For this review, take the finished solid that the model builds, in its own axes (mm). Face numbers are marked on the shaded views. Coordinates: 2 decimals unless noted, no trailing zeros. Return JSON: item names as keys, results as strings.
Autodesk Inventor part; units mm, degrees
ref_plane "YZ Plane" through (0, 0, 0) normal (1, 0, 0) x (0, 1, 0)
ref_plane "XZ Plane" through (0, 0, 0) normal (0, 1, 0) x (-1, 0, 0)
ref_plane "XY Plane" through (0, 0, 0) normal (0, 0, 1) x (1, 0, 0)
sketch "Sketch1" plane through (0, 0, 0) normal (0, 0, 1) x (1, 0, 0)
  circle A0 centre (0, 0) radius 23.15
  circle A1 centre (0, 0) radius 26.9875
  dimension "d0" = 46.3
  dimension "d1" = 53.975
extrude "Extrusion1" add sketch "Sketch1" along normal blind 12.7
chamfer "Chamfer1" distance 3.175 angle 45 1 edges at (-23.15, 0, 0)
sketch "Sketch2" plane through (0, 0, 0) normal (1, 0, 0) x (0, 1, 0)
  line L0 (26.9875, 0) -> (26.9875, 12.7)
  circle A0 centre (26.9875, 6.35) radius 1.5875
  line L1 (0, 0) -> (0, 25.7479) construction
  dimension "d7" = 3.175
revolve "Revolution1" cut sketch "Sketch2" angle 360 about axis through (0, 0, 0) along (0, 0, 1)
chamfer "Chamfer2" distance 1.5875 angle 45 1 edges at (-26.9875, 0, 12.7)
properties part number "Ring Hub" material "Nylon 6/6"
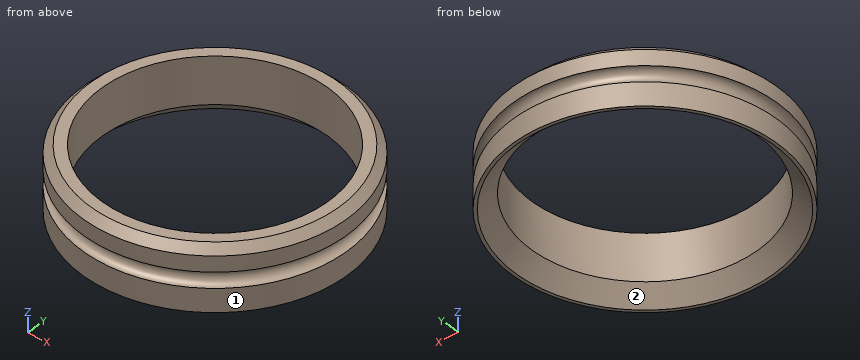
1. Clearance check with flat-ended pins moving along their axes: pin 1 Ø6 at (x, z) = (2, 2.5) entering from +Y; pin 2 Ø4 at (x, z) = (10.5, 7) entering from -Y; pin 3 Ø1.5 at (x, z) = (-15.5, 10.5) entering from +Y; pin 4 Ø1.5 at (y, z) = (-16.5, 6) entering from +X. State where each tip first meets the part, or that it passes through.
Checks:
{"pin 1": "y = 26.99", "pin 2": "y = -25.54", "pin 3": "y = 22.6", "pin 4": "x = 20.09"}
2. Draft analysis for pull direction X (two halves, no side actions). For the marked faces 1 and 2, state which applies: +X half, -X half, draft (parallel to the pull), parting line (faces both ways), or undercut.
Checks:
{"face 1": "parting line", "face 2": "undercut"}
3. Wall thickness on L1, parallel to Y at x = 0, z = 6.25; L2, parallel to Y at x = 0, z = 10; L3, parallel to X at y = -21, z = 5.25: over which ranges is each line inside the solid? List them lowest first. Write a range as from..to.
Checks:
{"L1": "-25.4..-23.15, 23.15..25.4", "L2": "-26.99..-23.15, 23.15..26.99", "L3": "-15.06..-9.74, 9.74..15.06"}
